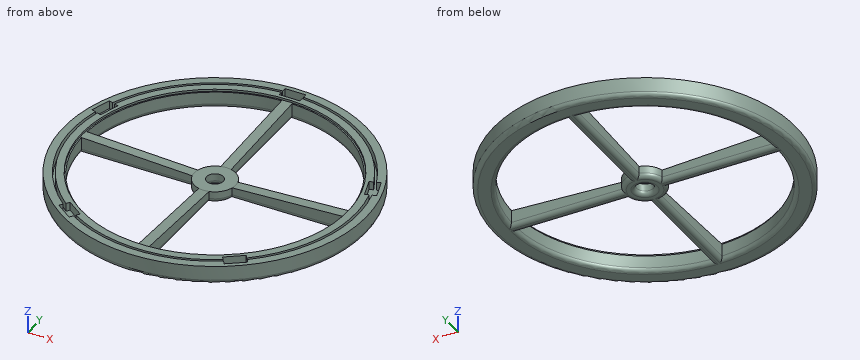
from build123d import *

# Parameters (mm, degrees)
F1_FACE1_R   = 80.9498
F1_FACE1_R_2 = 5.08
F3_DEPTH     = 25.4
F4_W         = 12.827
F4_H         = 6.731
F5_DEPTH     = 5.08
F10_R        = 2.54


with BuildPart() as f1:
    # F0 (on Front) → F1 (revolve)
    with BuildSketch(Plane.XZ):
        Polygon((80.9498, 0), (5.08, 0), (5.08, -10.16), (92.6526099873, -10.16), (92.6526099873, 1.27), (87.5726099873, 1.27), (87.5726099873, -3.81), (86.0298, -3.81), (86.0298, 1.27), (80.9498, 1.27), align=None)
    revolve(axis=Axis((0, 0, -1.5273375125), (0, 0, -1)))

    # F2 (on face) + F1_face1 (on face) → F3 (cut)
    with BuildSketch(Plane(origin=(0, 0, -10.16), x_dir=(1, 0, 0), z_dir=(0, 0, -1))):
        with BuildLine():
            Line((-3.175, 12.2967221242), (-3.175, 80.3791177001))
            ThreePointArc((-3.175, 80.3791177001), (-56.8809422709, 56.8809422709), (-80.3791177001, 3.175))
            Line((-80.3791177001, 3.175), (-12.2967221242, 3.175))
            ThreePointArc((-12.2967221242, 3.175), (-8.9802561211, 8.9802561211), (-3.175, 12.2967221242))
        make_face()
        with BuildLine():
            Line((-12.2967221242, -3.175), (-80.3791177001, -3.175))
            ThreePointArc((-80.3791177001, -3.175), (-56.8809422709, -56.8809422709), (-3.175, -80.3791177001))
            Line((-3.175, -80.3791177001), (-3.175, -12.2967221242))
            ThreePointArc((-3.175, -12.2967221242), (-8.9802561211, -8.9802561211), (-12.2967221242, -3.175))
        make_face()
        with BuildLine():
            Line((12.2967221242, 3.175), (80.3791177001, 3.175))
            ThreePointArc((80.3791177001, 3.175), (56.8809422709, 56.8809422709), (3.175, 80.3791177001))
            Line((3.175, 80.3791177001), (3.175, 12.2967221242))
            ThreePointArc((3.175, 12.2967221242), (8.9802561211, 8.9802561211), (12.2967221242, 3.175))
        make_face()
        with BuildLine():
            Line((3.175, -12.2967221242), (3.175, -80.3791177001))
            ThreePointArc((3.175, -80.3791177001), (56.8809422709, -56.8809422709), (80.3791177001, -3.175))
            Line((80.3791177001, -3.175), (12.2967221242, -3.175))
            ThreePointArc((12.2967221242, -3.175), (8.9802561211, -8.9802561211), (3.175, -12.2967221242))
        make_face()
    with BuildSketch(Plane.XY):
        Circle(F1_FACE1_R)
        Circle(F1_FACE1_R_2, mode=Mode.SUBTRACT)
    extrude(amount=-F3_DEPTH, dir=(0, 0, -1), mode=Mode.SUBTRACT)

    # F4 (on face) → F5 (cut)
    with BuildSketch(Plane.XY.offset(1.27)):
        with Locations((0, 86.5632)):
            Rectangle(F4_W, F4_H)
        Polygon((-83.5453956435, 33.8890975493), (-87.5091566304, 21.6898956148), (-81.1075952192, 19.6099022256), (-77.1438342323, 31.8091041602), align=None)
        Polygon((-58.0473941113, -68.9840858665), (-47.6701331244, -76.5236072976), (-43.7137505912, -71.0781139085), (-54.0910115781, -63.5385924773), align=None)
        Polygon((47.6701331244, -76.5236072976), (58.0473941113, -68.9840858665), (54.0910115781, -63.5385924773), (43.7137505912, -71.0781139085), align=None)
        Polygon((87.5091566304, 21.6898956148), (83.5453956435, 33.8890975493), (77.1438342323, 31.8091041602), (81.1075952192, 19.6099022256), align=None)
    extrude(amount=-F5_DEPTH, mode=Mode.SUBTRACT)


with BuildPart() as f6_1:
    # F6: copy of F1
    add(f1.part)


with BuildPart() as f1_1:
    add(f1.part)

    # F8 (on Front) → F9 (revolve, cut)
    with BuildSketch(Plane.XZ):
        Polygon((-81.28, 0), (-12.7, -3.175), (-3.4997510334, -3.175), (-4.5655716038, 5.7565840118), (-81.28, 5.608932225), align=None)
    revolve(axis=Axis((0, 0, -8.0116291065), (0, 0, -1)), mode=Mode.SUBTRACT)

    # F10
    f10_edges = [f1_1.edges().sort_by_distance(p)[0] for p in [
        (-92.65261, 0, -10.16),
        (3.175, 46.33792, -10.16),
        (8.980256, 8.980256, -10.16),
        (46.33792, 3.175, -10.16),
        (56.880942, 56.880942, -10.16),
        (-5.08, 0, -10.16),
        (-46.33792, 3.175, -10.16),
        (-8.980256, 8.980256, -10.16),
        (-3.175, 46.33792, -10.16),
        (-56.880942, 56.880942, -10.16),
        (46.33792, -3.175, -10.16),
        (8.980256, -8.980256, -10.16),
        (3.175, -46.33792, -10.16),
        (56.880942, -56.880942, -10.16),
        (-56.880942, -56.880942, -10.16),
        (-3.175, -46.33792, -10.16),
        (-8.980256, -8.980256, -10.16),
        (-46.33792, -3.175, -10.16),
    ]]
    fillet(f10_edges, radius=F10_R)


solid = f1_1.part
Could you check a few things on this model? Use its own coordinates, in mm. Coordinates: 2 decimals unless noted, no trailing zeros. Write each loop counter-clockwise with the first axis right and the second up, starting at its lowest first coordinate (ties: lowest second). Pieces come first, ordered by that corner, then holes. Notation, with made-up numbers: (37.25, 64.25) - (77.25, 64.25) arc R36 ccw to (77.25, 103.25) - close; hole circle Ø6 at (31, 15). An arc over 180 degrees is marked (long way). Put each result on its own line as item: value. Start each with the question number.
Q1. I want a section at A-A on z = -5.75. Write out the boundary of the cut face in (x, y) (3 decimals).
Q2. I'm going to push flat-ended pins straight in: P1, Ø0.8, axis at y = 84.5, z = -1, coming from the -X side; P2, Ø5, axis at y = -23.5, z = -7, coming from the +X side; P3, Ø4, axis at y = 62.5, z = -4, coming from the +X side. Where does each tip first touch, or does it pass through?
Q3. Please list where these lines run through material, in increasing order: L1, parallel to X at y = 0, z = -4.5; L2, parallel to Y at x = -25.5, z = -9; L3, parallel to X at y = 24.5, z = -3.75 (3 decimals).
Q4. I want a section at B-B on x = 15.5. Count the separate pieces of the cut face and the enclosed holes in it, plus the area to 3 significant figures.
Checks:
1. outline: circle Ø185.305 at (0, 0); hole (-80.379, -3.175) arc R80.442 ccw to (-3.175, -80.379) - (-3.175, -12.297) arc R12.7 cw to (-12.297, -3.175) - close; hole (-80.379, 3.175) - (-12.297, 3.175) arc R12.7 cw to (-3.175, 12.297) - (-3.175, 80.379) arc R80.442 ccw to start; hole circle Ø10.16 at (0, 0); hole (3.175, -80.379) arc R80.442 ccw to (80.379, -3.175) - (12.297, -3.175) arc R12.7 cw to (3.175, -12.297) - close; hole (3.175, 12.297) arc R12.7 cw to (12.297, 3.175) - (80.379, 3.175) arc R80.442 ccw to (3.175, 80.379) - close
2. P1: x = -38.88
2. P2: x = 90.24
2. P3: x = 70.17
3. L1: -92.65 to -5.08, 5.08 to 92.65
3. L2: -88.65 to -76.72, -2.77 to 2.77, 76.72 to 88.65
3. L3: -89.355 to -86.596, -79.519 to -76.62, -3.175 to 3.175, 76.62 to 79.519, 86.596 to 89.355
4. separate pieces: 3
4. enclosed holes: 0
4. area: 302 mm²
